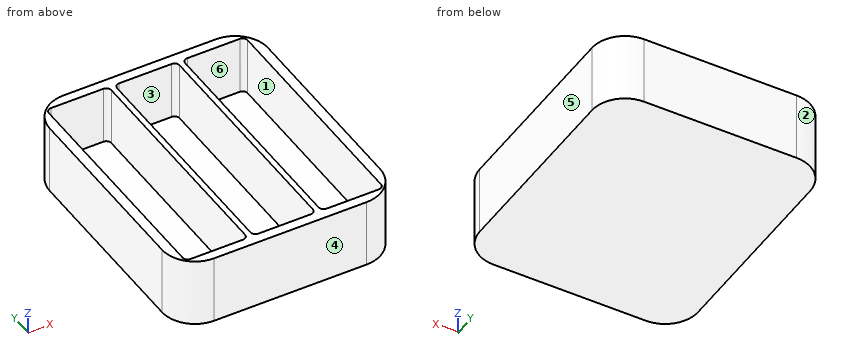
```python
from build123d import *

# Parameters (mm, degrees)
F0_W     = 279.4
F0_H     = 330.2
F1_DEPTH = 88.9
F2_R     = 42.251924
F4_DEPTH = 75.39211


with BuildPart() as f1:
    # F0 (on Top) → F1 (new body)
    with BuildSketch(Plane.XY):
        with Locations((139.7, -165.1)):
            Rectangle(F0_W, F0_H)
    extrude(amount=F1_DEPTH)

    # F2
    f2_edges = [f1.edges().sort_by_distance(p)[0] for p in [
        (0, -330.2, 44.45),
        (279.4, -330.2, 44.45),
        (279.4, 0, 44.45),
        (0, 0, 44.45),
    ]]
    fillet(f2_edges, radius=F2_R)

    # F3 (on face) → F4 (cut)
    with BuildSketch(Plane.XY.offset(88.9)):
        with BuildLine():
            ThreePointArc((99.771842, -311.15), (101.631714, -315.640128), (106.121842, -317.5))
            Line((106.121842, -317.5), (173.278158, -317.5))
            ThreePointArc((173.278158, -317.5), (177.768286, -315.640128), (179.628158, -311.15))
            Line((179.628158, -311.15), (179.628158, -19.05))
            ThreePointArc((179.628158, -19.05), (177.768286, -14.559872), (173.278158, -12.7))
            Line((173.278158, -12.7), (106.121842, -12.7))
            ThreePointArc((106.121842, -12.7), (101.631714, -14.559872), (99.771842, -19.05))
            Line((99.771842, -19.05), (99.771842, -311.15))
        make_face()
        with BuildLine():
            Line((260.35, -12.7), (193.193685, -12.7))
            ThreePointArc((193.193685, -12.7), (188.703557, -14.559872), (186.843685, -19.05))
            Line((186.843685, -19.05), (186.843685, -311.392798))
            ThreePointArc((186.843685, -311.392798), (188.703557, -315.882926), (193.193685, -317.742798))
            Line((193.193685, -317.742798), (260.35, -317.742798))
            ThreePointArc((260.35, -317.742798), (264.840128, -315.882926), (266.7, -311.392798))
            Line((266.7, -311.392798), (266.7, -19.05))
            ThreePointArc((266.7, -19.05), (264.840128, -14.559872), (260.35, -12.7))
        make_face()
        with BuildLine():
            Line((86.206315, -12.170881), (19.05, -12.170881))
            ThreePointArc((19.05, -12.170881), (14.559872, -14.030753), (12.7, -18.520881))
            Line((12.7, -18.520881), (12.7, -311.769943))
            ThreePointArc((12.7, -311.769943), (14.559872, -316.260071), (19.05, -318.119943))
            Line((19.05, -318.119943), (86.206315, -318.119943))
            ThreePointArc((86.206315, -318.119943), (90.696443, -316.260071), (92.556315, -311.769943))
            Line((92.556315, -311.769943), (92.556315, -18.520881))
            ThreePointArc((92.556315, -18.520881), (90.696443, -14.030753), (86.206315, -12.170881))
        make_face()
    extrude(amount=-F4_DEPTH, mode=Mode.SUBTRACT)


solid = f1.part
```
CAD build for the part. Positions are in the model's coordinates, mm. Face numbers are marked on the shaded views. A direction names the side the tool comes from. Round coordinates to 2 decimals unless told otherwise and drop trailing zeros. Write each loop counter-clockwise with the first axis right and the second up, starting at its lowest first coordinate (ties: lowest second). Pieces come first, ordered by that corner, then holes. Notation, with made-up numbers: (41.25, 66) - (90.25, 66) arc R23 cw to (90.25, 80) - close; hole circle Ø7 at (72.25, -38). An arc over 180 degrees is marked (long way). Return JSON: item names as keys, results as strings. Group by question number.
Item 1: Mould opens along X. For the marked faces 3, 4, 5 and 6 say: +X half, -X half, draft (parallel to the pull), parting line (faces both ways), or undercut.
Item 2: Band-saw the part on D-D on z = 7. List the corners of the cut face in (x, y).
Item 3: Flat gauge pins, fed straight in: pin 1 Ø6 at (x, y) = (72, -138.5) entering from +Z; pin 2 Ø1.5 at (y, z) = (-33, 36.5) entering from -X. Where does each tip first touch, or does it go through?
Item 4: Band-saw the part on B-B on y = -156. List the corners of the cut face in (x, z), plus the area to 3 significant figures.
Item 5: Band-saw the part on A-A on z = 57. State how many separate pieces and enclosed holes the cut face has, plus the area to 3 significant figures.
Item 6: Probe probe 1 along X at (y, z) = (-248.5, 58.5); probe 2 along X at (y, z) = (-294, 53.5); probe 3 along Y at (x, z) = (50.5, 82). List the from-to ranges inside material, lowest first.
Item 7: 3-axis set-ups, long thin cutter, end or side, ignore diameter. For the marked faces 1 and 2: which of +Z, -Z, +X, -X, +Y, -Y reach the whole face in a straight line?
Item 8: Band-saw the part on C-C on x = 226.5. List the corners of the cut face in (y, z).
Resolved:
{
 "1": {"face 3": "undercut", "face 4": "draft", "face 5": "+X half", "face 6": "undercut"},
 "2": {"outline": "(0, -287.95) arc R42.25 ccw to (42.25, -330.2) - (237.15, -330.2) arc R42.25 ccw to (279.4, -287.95) - (279.4, -42.25) arc R42.25 ccw to (237.15, 0) - (42.25, 0) arc R42.25 ccw to (0, -42.25) - close"},
 "3": {"pin 1": "stops at z = 13.51", "pin 2": "stops at x = 0.86"},
 "4": {"outline": "(0, 0) - (279.4, 0) - (279.4, 88.9) - (266.7, 88.9) - (266.7, 13.51) - (186.84, 13.51) - (186.84, 88.9) - (179.63, 88.9) - (179.63, 13.51) - (99.77, 13.51) - (99.77, 88.9) - (92.56, 88.9) - (92.56, 13.51) - (12.7, 13.51) - (12.7, 88.9) - (0, 88.9) - close", "area": "6,780 mm²"},
 "5": {"separate pieces": "1", "enclosed holes": "3", "area": "17,700 mm²"},
 "6": {"probe 1": "x = 0 to 12.7, 92.56 to 99.77, 179.63 to 186.84, 266.7 to 279.4", "probe 2": "x = 0.44 to 12.7, 92.56 to 99.77, 179.63 to 186.84, 266.7 to 278.96", "probe 3": "y = -330.2 to -318.12, -12.17 to 0"},
 "7": {"face 1": "+Z", "face 2": "+Z, -Z, -X, +Y"},
 "8": {"outline": "(-330.2, 0) - (0, 0) - (0, 88.9) - (-12.7, 88.9) - (-12.7, 13.51) - (-317.74, 13.51) - (-317.74, 88.9) - (-330.2, 88.9) - close"}
}
